Verification items for the finished model (mm, model axes). A direction names the side the tool comes from. Give positions to 0.01 mm unless a question says otherwise; leave off trailing zeros. Write each loop counter-clockwise with the first axis right and the second up, starting at its lowest first coordinate (ties: lowest second). Pieces come first, ordered by that corner, then holes. Notation, with made-up numbers: (30.25, 20) - (58.25, 20) arc R20 ccw to (58.25, 37) - close; hole circle Ø11 at (30.25, -2.75). An arc over 180 degrees is marked (long way). Put each result on its own line as item: value.
Autodesk Inventor part; units mm, degrees
ref_plane "YZ Plane" through (0, 0, 0) normal (1, 0, 0) x (0, 1, 0)
ref_plane "XZ Plane" through (0, 0, 0) normal (0, 1, 0) x (-1, 0, 0)
ref_plane "XY Plane" through (0, 0, 0) normal (0, 0, 1) x (1, 0, 0)
sketch "Sketch4" plane through (0, 0, 0) normal (0, 1, 0) x (-1, 0, 0)
  line L0 (-47.5, -47.5) -> (47.5, -47.5)
  line L1 (47.5, -47.5) -> (47.5, 47.5)
  line L2 (47.5, 47.5) -> (-47.5, 47.5)
  line L3 (-47.5, 47.5) -> (-47.5, -47.5)
  line L4 (-47.5, -47.5) -> (47.5, 47.5) construction
  line L5 (47.5, -47.5) -> (-47.5, 47.5) construction
  point P0 (0, 0)
  dimension "d24" = 95
  dimension "d25" = 95
extrude "Extrusion4" add sketch "Sketch4" along normal blind 5
sketch "Sketch5" plane through (0, 5, 0) normal (0, 1, 0) x (1, 0, 0)
  line L0 (-47.5, 47.5) -> (-47.5, -47.5)
  line L1 (-47.5, -42.5) -> (42.5, -42.5)
  line L2 (47.5, -47.5) -> (47.5, 47.5)
  line L3 (-47.5, -47.5) -> (47.5, -47.5)
  line L4 (42.5, -42.5) -> (42.5, 42.5)
  line L5 (-47.5, 42.5) -> (42.5, 42.5)
  line L6 (47.5, 47.5) -> (-47.5, 47.5)
  point P0 (0, 0)
  dimension "d28" = 5
  dimension "d29" = 5
  dimension "d30" = 5
extrude "Extrusion5" add sketch "Sketch5" along normal blind 25 contours L6 L2 L3 L0 L1 L4 L5
sketch "Sketch6" plane through (0, 30, 0) normal (0, 1, 0) x (1, 0, 0)
  circle A0 centre (45, -45) radius 1.6
  circle A1 centre (45, 45) radius 1.6
  line L0 (47.5, -47.5) -> (47.5, 47.5)
  line L1 (-47.5, -47.5) -> (47.5, -47.5)
  line L2 (47.5, 47.5) -> (-47.5, 47.5)
  point P0 (0, 0)
  dimension "d33" = 3.2
  dimension "d34" = 3.2
  dimension "d35" = 2.5
  dimension "d36" = 2.5
  dimension "d37" = 2.5
  dimension "d38" = 2.5
extrude "Extrusion6" cut sketch "Sketch6" against normal blind 25
sketch "Sketch7" plane through (47.5, 0, 47.5) normal (1, 0, 0) x (0, 0, -1)
  line L0 (39.95, 19.4) -> (55.05, 19.4)
  line L1 (55.05, 19.4) -> (55.05, 10.6)
  line L2 (55.05, 10.6) -> (39.95, 10.6)
  line L3 (39.95, 10.6) -> (39.95, 19.4)
  line L4 (39.95, 19.4) -> (55.05, 10.6) construction
  line L5 (55.05, 19.4) -> (39.95, 10.6) construction
  line L6 (0, 0) -> (95, 0)
  line L7 (0, 30) -> (95, 30)
  line L8 (0, 0) -> (0, 30)
  line L9 (95, 0) -> (95, 30)
  point P0 (47.5, 0)
  point P1 (47.5, 15)
  dimension "d41" = 15.1
  dimension "d42" = 8.8
  dimension "d43" = 10.6
  dimension "d44" = 10.6
  dimension "d45" = 39.95
  dimension "d46" = 39.95
extrude "Extrusion7" cut sketch "Sketch7" against normal blind 25 contours L0 L1 L2 L3
properties part number "Caja_Bateria"
Q1. Section check D-D, the plane z = -45. Record the cut outline in (x, y), plus the area to 3 significant figures.
Answers follow:
outline: (-47.5, 0) - (47.5, 0) - (47.5, 30) - (46.6, 30) - (46.6, 5) - (43.4, 5) - (43.4, 30) - (-47.5, 30) - close
area: 2,770 mm2
Q2. Set-up check for faces 1 (the face through (-3, 17, 42.5)), 2 (the face through (45, 15, 7.55)), 3 (the face through (1, 15, -47.5)), 4 (the face through (45, 5, -45)), 5 (the face through (-47.5, 4, 0)): record each of +Z, -Z, +X, -X, +Y, -Y from which the full face is reachable in a straight line by a thin tool's end or side.
Answers follow:
face 1: -X, +Y
face 2: +X, -X
face 3: -Z, +X, -X, +Y, -Y
face 4: +Y
face 5: +Z, -Z, -X, +Y, -Y
Q3. Section check A-A, the plane z = -6. Record the cut outline in (x, y), plus the area to 3 significant figures.
Answers follow:
outline: (-47.5, 0) - (47.5, 0) - (47.5, 10.6) - (42.5, 10.6) - (42.5, 5) - (-47.5, 5) - close; (42.5, 19.4) - (47.5, 19.4) - (47.5, 30) - (42.5, 30) - close
area: 556 mm2
Q4. Go/stop test with flat-tipped pins: pin 1 Ø8 at (x, z) = (35.5, 7) entering from -Y; pin 2 Ø12 at (x, z) = (35.5, 26) entering from +Y; pin 3 Ø7.5 at (y, z) = (14.5, 20.5) entering from -X; pin 4 Ø1.5 at (y, z) = (18.5, 3) entering from +X. Record where each tip stops, or that it passes through.
Answers follow:
pin 1: stops at y = 0
pin 2: stops at y = 5
pin 3: stops at x = 42.5
pin 4: passes through
Q5. Section check B-B, the plane x = 45. Record the cut outline in (y, z), plus the area to 3 significant figures.
Answers follow:
outline: (0, -47.5) - (30, -47.5) - (30, -46.6) - (5, -46.6) - (5, -43.4) - (30, -43.4) - (30, 43.4) - (5, 43.4) - (5, 46.6) - (30, 46.6) - (30, 47.5) - (0, 47.5) - close; hole (10.6, -7.55) - (19.4, -7.55) - (19.4, 7.55) - (10.6, 7.55) - close
area: 2,560 mm2
Q6. Release check for a two-part mould opening along X. For faces 6 (the face through (1, 0, 1)), 7 (the face through (45.74, 17.68, -43.58)), 8 (the face through (47.5, 8, 1)), 9 (the face through (45.74, 17.68, 46.42)) record: released by +X, released by -X, zero draft, split by the parting line, or undercut.
Answers follow:
face 6: zero draft
face 7: undercut
face 8: released by +X
face 9: undercut
Q7. Section check C-C, the plane y = 7.5. Record the cut outline in (x, z), plus the area to 3 significant figures.
Answers follow:
outline: (-47.5, -47.5) - (47.5, -47.5) - (47.5, 47.5) - (-47.5, 47.5) - (-47.5, 42.5) - (42.5, 42.5) - (42.5, -42.5) - (-47.5, -42.5) - close; hole circle Ø3.2 at (45, -45); hole circle Ø3.2 at (45, 45)
area: 1,360 mm2
Q8. Scan lines: line 1 along Z through (x, y) = (45, 21.25); line 2 along Z through (x, y) = (-37.5, 21.5); line 3 along X through (y, z) = (16.5, 45). Record each from-to range of solid material in increasing order.
Answers follow:
line 1: z = -47.5 to -46.6, -43.4 to 43.4, 46.6 to 47.5
line 2: z = -47.5 to -42.5, 42.5 to 47.5
line 3: x = -47.5 to 43.4, 46.6 to 47.5
